Study the drawing (mm; zero at the part's minimum x, y, z) and answer. Coordinates: 2 decimals unless noted, no trailing zeros. Write each loop counter-clockwise with the first axis right and the second up, starting at its lowest first coordinate (ties: lowest second). Pieces come first, ordered by that corner, then holes. Notation, with made-up numbers: (-2.5, -28.75) -> (8.5, -28.75) arc R14 cw to (8.5, -12.75) -> close; hole circle Ø5 at (89.5, 54.25). An arc over 180 degrees is marked (long way). Write each question's results on one line, items separated by ' | '. Start each with the question number.
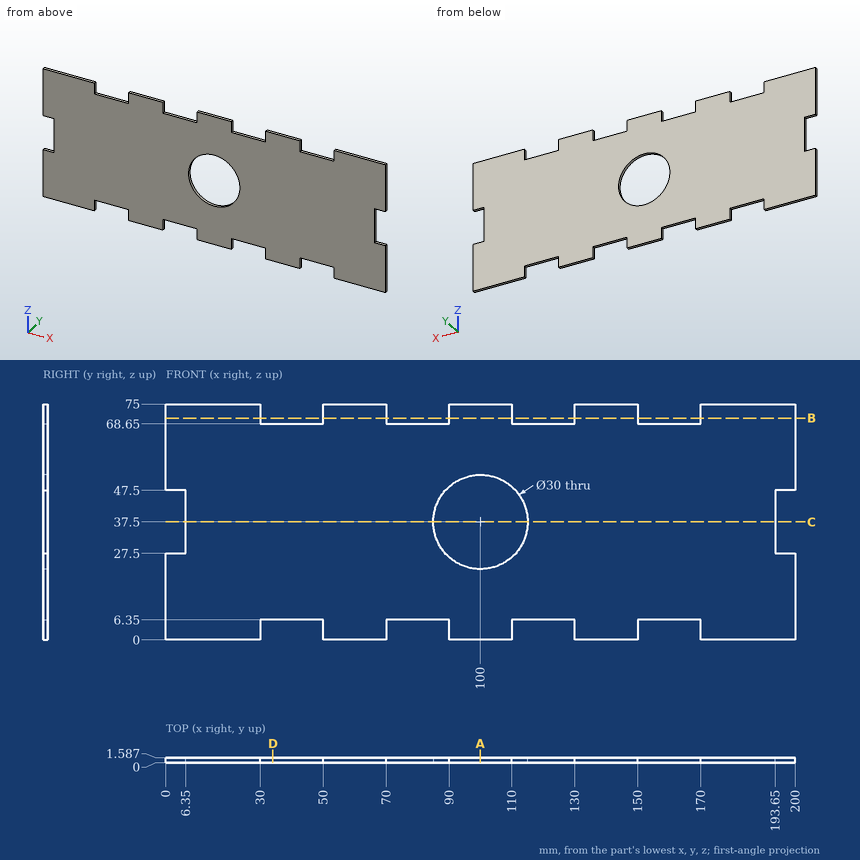
1. Find the intervals of material crossed by L1, parallel to X at y = 0.9, z = 69; L2, parallel to X at y = 0.5, z = 37.5; L3, parallel to Z at x = 100, y = 1, in increasing order.
2. Find section C-C on z = 37.5. Give the vertices of the cut face in (x, y).
3. Find section D-D on x = 34. Give the vertices of the cut face in (y, z).
4. Find section B-B on z = 70.5. Give the vertices of the cut face in (x, y).
5. Find section A-A on x = 100. Give the vertices of the cut face in (y, z).
6. Given pin 1 Ø0.5 at (y, z) = (1, 35.5) entering from +X; pin 2 Ø0.8 at (x, y) = (83.5, 0.5) entering from -Z; pin 3 Ø0.8 at (x, y) = (84, 1) entering from +Z, each flat-ended and moving along its own axis, determine where each tip first touches the part or whether it passes through.
Ans:
1) L1: x = 0 to 30, 50 to 70, 90 to 110, 130 to 150, 170 to 200 | L2: x = 6.35 to 85, 115 to 193.65 | L3: z = 0 to 22.5, 52.5 to 75
2) outline: (6.35, 0) -> (85, 0) -> (85, 1.59) -> (6.35, 1.59) -> close; (115, 0) -> (193.65, 0) -> (193.65, 1.59) -> (115, 1.59) -> close
3) outline: (0, 6.35) -> (1.59, 6.35) -> (1.59, 68.65) -> (0, 68.65) -> close
4) outline: (0, 0) -> (30, 0) -> (30, 1.59) -> (0, 1.59) -> close; (50, 0) -> (70, 0) -> (70, 1.59) -> (50, 1.59) -> close; (90, 0) -> (110, 0) -> (110, 1.59) -> (90, 1.59) -> close; (130, 0) -> (150, 0) -> (150, 1.59) -> (130, 1.59) -> close; (170, 0) -> (200, 0) -> (200, 1.59) -> (170, 1.59) -> close
5) outline: (0, 0) -> (1.59, 0) -> (1.59, 22.5) -> (0, 22.5) -> close; (0, 52.5) -> (1.59, 52.5) -> (1.59, 75) -> (0, 75) -> close
6) pin 1: stops at x = 193.65 | pin 2: stops at z = 6.35 | pin 3: stops at z = 68.65
